The listing builds one solid part. Answer for the finished solid, in the listing's coordinates (mm). A direction names the side the tool comes from. Give positions to 0.01 mm unless a question says otherwise; leave off trailing zeros. Write each loop counter-clockwise with the first axis right and the second up, starting at its lowest first coordinate (ties: lowest second). Pieces come first, ordered by that corner, then holes. Notation, with made-up numbers: (14.5, -4.75) - (43.5, -4.75) arc R22 ccw to (43.5, 28.25) - close; hole circle Ø6 at (-9, 66.25). An arc over 180 degrees is marked (long way). One line per item, written item: value. Start each with the question number.
from build123d import *

# Parameters (mm, degrees)
RESSALTO_EXTRUS_O1_DEPTH = 50
ESBO_O2_W                = 6
ESBO_O2_H                = 2
CORTE_EXTRUS_O1_DEPTH    = 10
ESBO_O3_W                = 6
ESBO_O3_H                = 20
CORTE_EXTRUS_O2_DEPTH    = 2
FILETE1_R                = 3


with BuildPart() as part:
    # Esboço1 → Ressalto-extrusão1 (new body)
    with BuildSketch(Plane.XY):
        with BuildLine():
            Line((0, 35), (0, -35))
            Line((0, -35), (13.5, -35))
            Line((13.5, -35), (13.5, -32.5))
            ThreePointArc((13.5, -32.5), (6, -25), (13.5, -17.5))
            Line((13.5, -17.5), (13.5, -15))
            Line((13.5, -15), (6, -15))
            Line((6, -15), (6, 15))
            Line((6, 15), (13.5, 15))
            Line((13.5, 15), (13.5, 17.5))
            ThreePointArc((13.5, 17.5), (6, 25), (13.5, 32.5))
            Line((13.5, 32.5), (13.5, 35))
            Line((13.5, 35), (0, 35))
        make_face()
    extrude(amount=RESSALTO_EXTRUS_O1_DEPTH)

    # Esboço2 → Corte-extrusão1 (cut)
    with BuildSketch(Plane(origin=(6, 0, 0), x_dir=(0, 0, -1), z_dir=(1, 0, 0))):
        with Locations((-10, 14)):
            Rectangle(ESBO_O2_W, ESBO_O2_H)
        with Locations((-40, 14)):
            Rectangle(ESBO_O2_W, ESBO_O2_H)
        with Locations((-40, -14)):
            Rectangle(ESBO_O2_W, ESBO_O2_H)
        with Locations((-10, -14)):
            Rectangle(ESBO_O2_W, ESBO_O2_H)
    extrude(amount=-CORTE_EXTRUS_O1_DEPTH, mode=Mode.SUBTRACT)

    # Esboço3 → Corte-extrusão2 (cut)
    with BuildSketch(Plane.ZY):
        with Locations((10, 25)):
            Rectangle(ESBO_O3_W, ESBO_O3_H)
        with Locations((40, 25)):
            Rectangle(ESBO_O3_W, ESBO_O3_H)
        with Locations((40, -25)):
            Rectangle(ESBO_O3_W, ESBO_O3_H)
        with Locations((10, -25)):
            Rectangle(ESBO_O3_W, ESBO_O3_H)
    extrude(amount=-CORTE_EXTRUS_O2_DEPTH, mode=Mode.SUBTRACT)

    # Filete1
    filete1_edges = [part.edges().sort_by_distance(p)[0] for p in [
        (2, 15, 10),
        (2, 35, 10),
        (2, 15, 40),
        (2, 35, 40),
        (2, -15, 40),
        (2, -35, 40),
        (2, -15, 10),
        (2, -35, 10),
    ]]
    fillet(filete1_edges, radius=FILETE1_R)


solid = part.part
Item 1: For faces 1 (the flat face through (3, 13, 10)), 2 (the flat face through (6, 0, 25)), 3 (the flat face through (1.6, 21.4, 43)), 4 (the cylindrical face through (2.86, 34.1, 40.04)), determine the directions among +Z, -Z, +X, -X, +Y, -Y from which every point of the face is accessible in a straight line to the end or side of a thin tool.
Item 2: Straight lines are drawn through the part: line 1 along Z through (x, y) = (1.75, 14); line 2 along Y through (x, z) = (5.5, 10); line 3 along Y through (x, z) = (11.5, 21.5). For each, find the intervals that lie inside material, in ascending order.
Item 3: Each of these flat-tipped pins is pushed along its axis until it touches: pin 1 Ø6.5 at (x, y) = (2.5, -21) entering from -Z; pin 2 Ø15 at (y, z) = (0.5, 36.5) entering from +X; pin 3 Ø5 at (x, y) = (9, -4.5) entering from +Z; pin 4 Ø2 at (x, z) = (2, 40) entering from +Y. Where does it stop, or does it pass through?
Item 4: Find section A-A on x = 7.5. Determine the outline of the cut face in (y, z).
Item 5: Find section B-B on y = 25. Determine the outline of the cut face in (x, z).
Item 6: Find section D-D on y = 10.5. Determine the outline of the cut face in (x, z), plus the area to 3 significant figures.
Item 7: Find section C-C on x = 1. Determine the outline of the cut face in (y, z), plus the area to 3 significant figures.
Item 8: The mould has two halves that part along Z. Classify faces 5 (the flat face through (7, -35, 25)), 6 (the flat face through (2, -25, 40)): +Z half, -Z half, draft (parallel to the pull), parting line (faces both ways), or undercut.
Values:
1. face 1: +X, -X
1. face 2: +Z, -Z, +X
1. face 3: -X
1. face 4: -X, +Y
2. line 1: 0 to 7, 13 to 37, 43 to 50
2. line 2: -35 to -15, -13 to 13, 15 to 35
2. line 3: -35 to -32.23, -17.77 to -15, 15 to 17.77, 32.23 to 35
3. pin 1: z = 0
3. pin 2: x = 6
3. pin 3: through
3. pin 4: y = 34.24
4. outline: (-35, 0) - (-29.5, 0) - (-29.5, 50) - (-35, 50) - close; (-20.5, 0) - (-15, 0) - (-15, 50) - (-20.5, 50) - close; (15, 0) - (20.5, 0) - (20.5, 50) - (15, 50) - close; (29.5, 0) - (35, 0) - (35, 50) - (29.5, 50) - close
5. outline: (0, 0) - (6, 0) - (6, 50) - (0, 50) - (0, 43) - (2, 43) - (2, 37) - (0, 37) - (0, 13) - (2, 13) - (2, 7) - (0, 7) - close
6. outline: (0, 0) - (6, 0) - (6, 50) - (0, 50) - close
6. area: 300 mm^2
7. outline: (-35, 0) - (35, 0) - (35, 7) - (13, 7) - (13, 13) - (35, 13) - (35, 37) - (13, 37) - (13, 43) - (35, 43) - (35, 50) - (-35, 50) - (-35, 43) - (-13, 43) - (-13, 37) - (-35, 37) - (-35, 13) - (-13, 13) - (-13, 7) - (-35, 7) - close
7. area: 2,970 mm^2
8. face 5: draft
8. face 6: undercut
